For this review, take the finished solid that the model builds, in its own axes (mm). Face numbers are marked on the shaded views. A direction names the side the tool comes from. Give positions to 0.01 mm unless a question says otherwise; leave off trailing zeros. Order: outer loops, then holes, each group sorted by start corner. A loop starts at its lowest first (then second) coordinate and runs counter-clockwise, first axis right, second up. Notation, with made-up numbers: (-22.5, 60.25) - (4.5, 60.25) arc R17 cw to (4.5, 93.25) - close; hole circle Ø11 at (69.5, -25). An arc over 180 degrees is marked (long way). Answer as a JSON object with one key per item and string values. Group by question number.
from build123d import *

# Parameters (mm, degrees)
F0_W      = 29
F0_H      = 16.5
F1_DEPTH  = 38.5
F2_T      = -2
F3_DEPTH  = 2.25
F4_SIZE   = 2
F5_SIZE   = 0.99999
F7_DEPTH  = 16.501
F9_DEPTH  = 2
F10_R     = 2
F11_DEPTH = 2.001
F12_W     = 7.54
F12_H     = 7.25
F12_R     = 1.1
F13_DEPTH = 6.35
F14_W     = 5.538
F14_H     = 5.533
F16_W     = 5.538
F16_H     = 4.583


# Not quite as in the source:
# - a fillet or chamfer is up to 0.001 mm smaller than in the source, because OpenCascade refuses the exact size


with BuildPart() as f1:
    # F0 (on Top) → F1 (new body)
    with BuildSketch(Plane.XY):
        with Locations((14.5, 8.25)):
            Rectangle(F0_W, F0_H)
    extrude(amount=F1_DEPTH)

    # F2
    f2_openings = [f1.faces().sort_by_distance(p)[0] for p in [
        (14.5, 8.25, 38.5),
    ]]
    offset(amount=F2_T, openings=f2_openings)

    # F3 (add): a face of the model
    f3_faces = [f1.faces().sort_by_distance(p)[0] for p in [
        (14.5, 8.25, 2),
    ]]
    extrude(f3_faces, amount=F3_DEPTH)

    # F4
    f4_edges = [f1.edges().sort_by_distance(p)[0] for p in [
        (0, 16.5, 19.25),
        (0, 0, 19.25),
        (29, 16.5, 19.25),
        (29, 0, 19.25),
        (14.5, 16.5, 0),
        (14.5, 0, 0),
        (29, 8.25, 0),
        (0, 8.25, 0),
    ]]
    chamfer(f4_edges, length=F4_SIZE)

    # F5 (size 1 in the source; OpenCascade refuses exactly that, so slightly less here)
    f5_edges = [f1.edges().sort_by_distance(p)[0] for p in [
        (14.5, 16.5, 38.5),
        (14.5, 0, 38.5),
        (0, 8.25, 38.5),
        (29, 8.25, 38.5),
    ]]
    chamfer(f5_edges, length=F5_SIZE)

    # F6 (on face) → F7 (cut, through all)
    with BuildSketch(Plane.XZ):
        Polygon((6.464, 8.664), (6.464, 4.94), (23.536, 4.94), (23.536, 8.664), (17.364, 12.834), (12.635, 12.834), align=None)
    extrude(amount=-F7_DEPTH, mode=Mode.SUBTRACT)

    # F8 (on face) → F9 (cut, through all)
    with BuildSketch(Plane.YZ.offset(29)):
        with BuildLine():
            Line((14.5, 38.5), (2, 38.5))
            Line((2, 38.5), (2, 28.5))
            ThreePointArc((2, 28.5), (8.25, 34.75), (14.5, 28.5))
            Line((14.5, 28.5), (14.5, 38.5))
        make_face()
        with BuildLine():
            ThreePointArc((14.5, 28.5), (8.25, 34.75), (2, 28.5))
            Line((2, 28.5), (14.5, 28.5))
        make_face()
        with BuildLine():
            Line((14.5, 28.5), (2, 28.5))
            ThreePointArc((2, 28.5), (2.8024937382, 25.4361502113), (5.0038961688, 23.1590909091))
            ThreePointArc((5.0038961688, 23.1590909091), (8.25, 26.25), (11.4961038312, 23.1590909091))
            ThreePointArc((11.4961038312, 23.1590909091), (13.6975062618, 25.4361502113), (14.5, 28.5))
        make_face()
        with BuildLine():
            ThreePointArc((11.4961038312, 23.1590909091), (8.25, 26.25), (5.0038961688, 23.1590909091))
            ThreePointArc((5.0038961688, 23.1590909091), (8.25, 22.25), (11.4961038312, 23.1590909091))
        make_face()
        with BuildLine():
            ThreePointArc((11.4961038312, 23.1590909091), (8.25, 22.25), (5.0038961688, 23.1590909091))
            ThreePointArc((5.0038961688, 23.1590909091), (8.1704306945, 19.7509741882), (11.5, 23))
            ThreePointArc((11.5, 23), (11.4990258118, 23.0795693055), (11.4961038312, 23.1590909091))
        make_face()
    extrude(amount=-F9_DEPTH, mode=Mode.SUBTRACT)

    # F10 (on face) → F11 (cut, through all)
    with BuildSketch(Plane.YZ.offset(2)):
        with Locations((8.25, 23)):
            Circle(F10_R)
    extrude(amount=-F11_DEPTH, mode=Mode.SUBTRACT)

    # F12 (on face) → F13 (join)
    with BuildSketch(Plane.YZ.offset(29)):
        with Locations((8.25, 7.875)):
            Rectangle(F12_W, F12_H)
        with Locations((8.25, 9)):
            Circle(F12_R, mode=Mode.SUBTRACT)
    extrude(amount=-F13_DEPTH)

    # F14 (on face) → F17 section 0
    with BuildSketch(Plane.YZ.offset(29)):
        with Locations((8.25, 8.0385)):
            Rectangle(F14_W, F14_H)
    # F16 (on offset) → F17 section 1
    with BuildSketch(Plane.YZ.offset(24.55)):
        with Locations((8.25, 8.5135)):
            Rectangle(F16_W, F16_H)
    loft(mode=Mode.SUBTRACT)


solid = f1.part
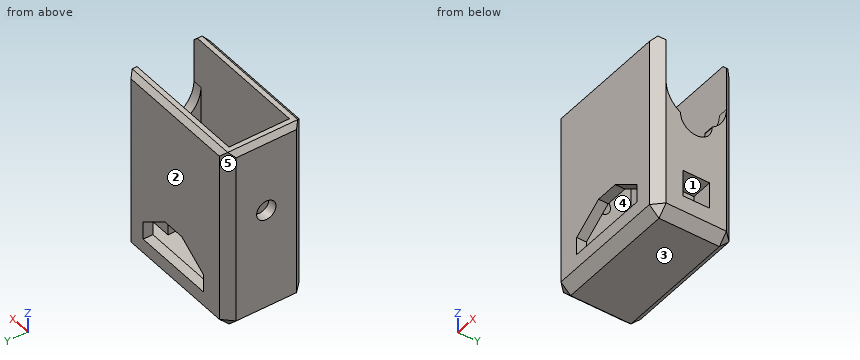
1) Consider section D-D (z = 30). Give the boundary of the cut face in (x, y), plus the area to 3 significant figures.
2) For line 1 (Y direction, x = 7.5, z = 28); line 2 (X direction, y = 3.5, z = 21.5); line 3 (Z direction, x = 24, y = 8.25), list the stretches that pass through material, from the lowest coordinate up.
3) Mouldability with a two-part tool opening along Z and no side actions: class the marked faces 1, 2 and 3 as released by +Z, released by -Z, zero draft, split by the parting line, or undercut.
4) Consider section A-A (y = 8.25). Give the boundary of the cut face in (x, z) (3 decimals).
5) Consider section B-B (x = 9). Give the boundary of the cut face in (y, z).
6) Consider section C-C (x = 4.5). Give the boundary of the cut face in (y, z).
7) For pin 1 (0.6 mm diameter, centred on y = 1, z = 6, fed in from -X); pin 2 (0.6 mm diameter, centred on y = 0.5, z = 6, fed in from +X); pin 3 (2.5 mm diameter, centred on y = 8.5, z = 8, fed in from +X), all flat-tipped, find the tip position at first contact; note any pin that passes through.
8) For the marked faces 4 and 5, list the 3-axis set-ups (+Z, -Z, +X, -X, +Y, -Y) from which the entire face can be reached by the end or side of a thin tool; tool diameter is ignored.
Result set:
{
 "1": {"outline": "(0, 2) - (2, 0) - (27, 0) - (29, 2) - (2, 2) - (2, 14.5) - (29, 14.5) - (27, 16.5) - (2, 16.5) - (0, 14.5) - close", "area": "133 mm2"},
 "2": {"line 1": "y = 0 to 2, 14.5 to 16.5", "line 2": "x = 0 to 2, 27 to 29", "line 3": "z = 0 to 7.9, 10.1 to 11.5"},
 "3": {"face 1": "undercut", "face 2": "zero draft", "face 3": "released by -Z"},
 "4": {"outline": "(0, 2) - (2, 0) - (27, 0) - (29, 2) - (29, 5.272) - (24.55, 6.222) - (24.55, 7.9) - (22.65, 7.9) - (22.65, 4.25) - (2, 4.25) - (2, 21) - (0, 21) - close; (0, 25) - (2, 25) - (2, 38.5) - (1, 38.5) - (0, 37.5) - close; (22.65, 10.1) - (24.55, 10.1) - (24.55, 10.805) - (29, 10.805) - (29, 19.75) - (27, 19.75) - (27, 11.5) - (22.65, 11.5) - close"},
 "5": {"outline": "(0, 2) - (2, 0) - (14.5, 0) - (16.5, 2) - (16.5, 4.94) - (14.5, 4.94) - (14.5, 4.25) - (2, 4.25) - (2, 4.94) - (0, 4.94) - close; (0, 10.38) - (2, 10.38) - (2, 38.5) - (1, 38.5) - (0, 37.5) - close; (14.5, 10.38) - (16.5, 10.38) - (16.5, 37.5) - (15.5, 38.5) - (14.5, 38.5) - close"},
 "6": {"outline": "(0, 2) - (2, 0) - (14.5, 0) - (16.5, 2) - (16.5, 37.5) - (15.5, 38.5) - (14.5, 38.5) - (14.5, 4.25) - (2, 4.25) - (2, 38.5) - (1, 38.5) - (0, 37.5) - close"},
 "7": {"pin 1": "stops at x = 0.7", "pin 2": "stops at x = 27.8", "pin 3": "stops at x = 24.55"},
 "8": {"face 4": "+Z", "face 5": "+Z, -Z, -X, +Y"}
}
